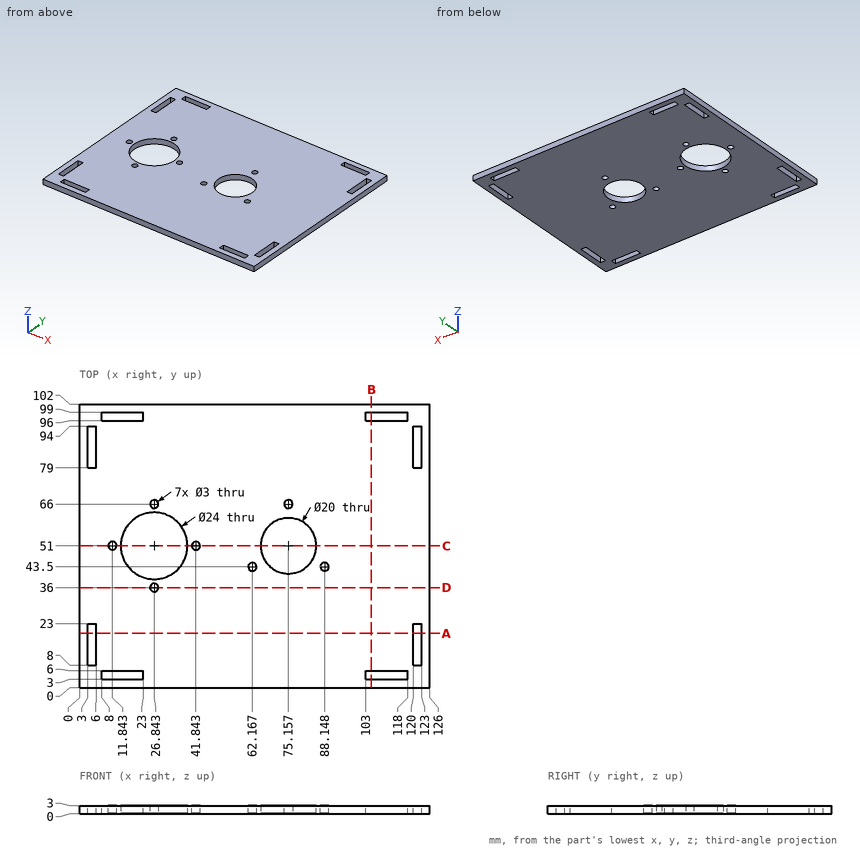
Here's the drawing with two shaded views (mm, measured from the low corner). I have some questions. Coordinates: 2 decimals unless noted, no trailing zeros. Write each loop counter-clockwise with the first axis right and the second up, starting at its lowest first coordinate (ties: lowest second). Pieces come first, ordered by that corner, then holes. Notation, with made-up numbers: (-39, -3.5) -> (7, -3.5) arc R24 cw to (7, 33.5) -> close; hole circle Ø10 at (24.25, 11). An arc over 180 degrees is marked (long way). Write item = value, one per line. Start each with the question number.
(1) I want a section at D-D (y = 36). Please give me the cut outline in (x, z).
(2) I want a section at A-A (y = 19.5). Please give me the cut outline in (x, z).
(3) I need wall thicknesses on line 1 (Y direction, x = 10, z = 2.65); line 2 (X direction, y = 81.5, z = 1.25); line 3 (Y direction, x = 27, z = 2.5). Which ranges of each line are inside material? Lowest first, please. Write a range as [from, to].
(4) Will this pin go through, and if not, where does the flat tip stop? pin 1 (23 mm diameter, centred on x = 75.16, y = 51, fed in from -Z).
(5) I want a section at C-C (y = 51). Please give me the cut outline in (x, z), plus the area to 3 significant figures.
(6) I want a section at B-B (x = 105). Please give me the cut outline in (y, z), plus the area to 3 significant figures.
Result set:
q1.outline = (0, 0) -> (25.34, 0) -> (25.34, 3) -> (0, 3) -> close; (28.34, 0) -> (126, 0) -> (126, 3) -> (28.34, 3) -> close
q2.outline = (0, 0) -> (3, 0) -> (3, 3) -> (0, 3) -> close; (6, 0) -> (120, 0) -> (120, 3) -> (6, 3) -> close; (123, 0) -> (126, 0) -> (126, 3) -> (123, 3) -> close
q3.line_1 = [0, 3], [6, 96], [99, 102]
q3.line_2 = [0, 3], [6, 120], [123, 126]
q3.line_3 = [0, 34.51], [37.49, 39], [63, 64.51], [67.49, 102]
q4.pin_1 = 0
q5.outline = (0, 0) -> (10.34, 0) -> (10.34, 3) -> (0, 3) -> close; (13.34, 0) -> (14.84, 0) -> (14.84, 3) -> (13.34, 3) -> close; (38.84, 0) -> (40.34, 0) -> (40.34, 3) -> (38.84, 3) -> close; (43.34, 0) -> (65.16, 0) -> (65.16, 3) -> (43.34, 3) -> close; (85.16, 0) -> (126, 0) -> (126, 3) -> (85.16, 3) -> close
q5.area = 228 mm2
q6.outline = (0, 0) -> (3, 0) -> (3, 3) -> (0, 3) -> close; (6, 0) -> (96, 0) -> (96, 3) -> (6, 3) -> close; (99, 0) -> (102, 0) -> (102, 3) -> (99, 3) -> close
q6.area = 288 mm2
